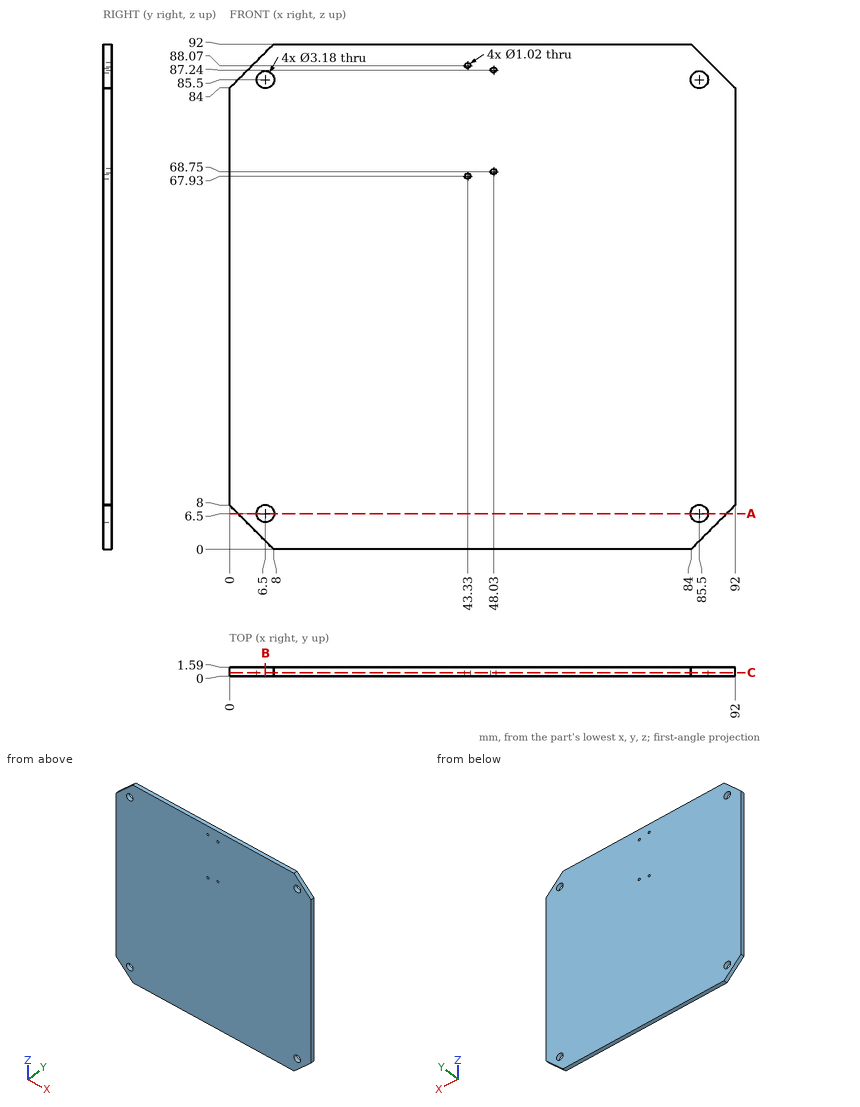
Can you work these out from the drawing? Everything is in mm from the part's minimum corner. Give positions to 0.01 mm unless a question says otherwise; leave off trailing zeros. Order: outer loops, then holes, each group sorted by start corner. A loop starts at its lowest first (then second) coordinate and runs counter-clockwise, first axis right, second up.
Item 1: If we section it at B-B, the plane x = 6.5: Write out the boundary of the cut face in (y, z), plus the area to 3 significant figures.
Item 2: If we section it at A-A, the plane z = 6.5: Write out the boundary of the cut face in (x, y).
Item 3: If we section it at C-C, the plane y = 0.6: Count the separate pieces of the cut face and the enclosed holes in it, plus the area to 3 significant figures.
Item 4: I need wall thicknesses on line 1 (Z direction, x = 43.33, y = 1.2); line 2 (X direction, y = 1, z = 85.5); line 3 (X direction, y = 0.5, z = 67.93). Which ranges of each line are inside material? Lowest first, please.
Item 5: I'm going to push a flat-ended pin straight in: pin 1 (5 mm diameter, centred on x = 85.5, z = 6.5, fed in from -Y). Where does the tip first touch, or does it pass through?
Values:
1. outline: (0, 1.5) - (1.59, 1.5) - (1.59, 4.91) - (0, 4.91) - close; (0, 8.09) - (1.59, 8.09) - (1.59, 83.91) - (0, 83.91) - close; (0, 87.09) - (1.59, 87.09) - (1.59, 90.5) - (0, 90.5) - close
1. area: 131 mm2
2. outline: (1.5, 0) - (4.91, 0) - (4.91, 1.59) - (1.5, 1.59) - close; (8.09, 0) - (83.91, 0) - (83.91, 1.59) - (8.09, 1.59) - close; (87.09, 0) - (90.5, 0) - (90.5, 1.59) - (87.09, 1.59) - close
3. separate pieces: 1
3. enclosed holes: 8
3. area: 8,300 mm2
4. line 1: z = 0 to 67.42, 68.44 to 87.56, 88.58 to 92
4. line 2: x = 1.5 to 4.91, 8.09 to 83.91, 87.09 to 90.5
4. line 3: x = 0 to 42.82, 43.84 to 92
5. pin 1: stops at y = 0
